Here's how the part is built. I have some questions about the finished solid (model axes, mm). A direction names the side the tool comes from. Round coordinates to 2 decimals unless told otherwise and drop trailing zeros. Order: outer loops, then holes, each group sorted by start corner. A loop starts at its lowest first (then second) coordinate and runs counter-clockwise, first axis right, second up.
Autodesk Inventor part; units mm, degrees
ref_plane "YZ Plane" through (0, 0, 0) normal (1, 0, 0) x (0, 1, 0)
ref_plane "XZ Plane" through (0, 0, 0) normal (0, 1, 0) x (-1, 0, 0)
ref_plane "XY Plane" through (0, 0, 0) normal (0, 0, 1) x (1, 0, 0)
sketch "スケッチ1" plane through (0, 0, 0) normal (1, 0, 0) x (0, 1, 0)
  circle A0 centre (0, 0) radius 9
  line L0 (50, 5.5) -> (-9, 5.5)
  line L1 (-9, 5.5) -> (-9, -13.5)
  line L2 (-9, -13.5) -> (50, -13.5)
  line L3 (50, -13.5) -> (50, 5.5)
  line L4 (50, 13.5) -> (-9, 13.5)
  line L5 (-9, 13.5) -> (-9, -13.5)
  line L6 (-9, -13.5) -> (50, -13.5)
  line L7 (50, -13.5) -> (50, 13.5)
  line L8 (-20.8, 0) -> (61.8, 0)
  point P0 (-9, 0)
  dimension "d0" = 18
  dimension "d3" = 19
  dimension "d4" = 27
extrude "押し出し1" add sketch "スケッチ1" along normal blind 1.5 contours L8 L3 L2 L1 A0 | A0 L0 L3 L8 | L1 L0 A0
sketch "スケッチ2" plane through (0, 0, 0) normal (-1, 0, 0) x (0, 0, 1)
  arc A0 (-0.2778, 12.9845) -> (-2.4907, 10.2851) centre (0, 10.5) ccw
  line L0 (-3.4833, 8.3812) -> (-3.5, 8.3716)
  line L1 (-3.5, 8.3716) -> (-3.5, 20)
  line L2 (-3.5, 20) -> (-0.5, 20)
  line L3 (-7, 20) -> (-3.5, 20)
  arc A1 (-4.5, 7.7942) -> (-5.7273, 6.9425) centre (0, 0) ccw
  line L4 (-3.5, 8.3716) -> (-4.5, 7.7942)
  arc A2 (5.5, 7.1239) -> (0, -9) centre (0, 0) ccw
  line L5 (5.5, 50) -> (5.5, 7.1239)
  line L6 (-13.5, 50) -> (5.5, 50)
  line L7 (-13.5, -9) -> (-13.5, 50)
  line L8 (0, -9) -> (-13.5, -9)
  line L9 (5.5, -9) -> (0, -9)
  line L10 (5.5, -7.1239) -> (5.5, -9)
  arc A3 (0, -9) -> (5.5, -7.1239) centre (0, 0) ccw
  arc A4 (-3.4833, 8.3812) -> (-2.4907, 10.2851) centre (-4.4833, 10.1132) ccw
  arc A5 (1.5, 18) -> (-0.5, 20) centre (-0.5, 18) ccw
  line L11 (1.5, 18) -> (1.5, 14.9721)
  arc A6 (-0.2778, 12.9845) -> (1.5, 14.9721) centre (-0.5, 14.9721) ccw
  line L12 (-9, 8.4853) -> (-9, 18)
  arc A7 (-7, 20) -> (-9, 18) centre (-7, 18) ccw
  arc A8 (-9, 8.4853) -> (-5.7273, 6.9425) centre (-7, 8.4853) ccw
  point P0 (-4.5, 7.7942)
  point P1 (-5.7273, 6.9425)
extrude "押し出し2" cut sketch "スケッチ2" against normal through all contours A6 L11 A5 L2 L3 A7 L12 A8 A2 L8 L7 L6 L5 L4 L0 A4 A0 | A3 L10 L9
sketch "スケッチ3" plane through (0, 0, 0) normal (-1, 0, 0) x (0, 0, 1)
  line L0 (-3.5, 20) -> (-3.5, 8.3716)
  line L1 (-4.5, 7.7942) -> (-3.4833, 8.3812)
  arc A0 (-0.2778, 12.9845) -> (-2.4907, 10.2851) centre (0, 10.5) ccw
  line L2 (-0.5, 20) -> (-7, 20)
  arc A1 (-4.5, 7.7942) -> (-5.7273, 6.9425) centre (0, 0) ccw
  line L3 (-3.5, 20) -> (-2.5, 20)
  line L4 (-2.5, 20) -> (-2.5, 8.3716)
  line L5 (-2.5, 8.3716) -> (-3.5, 8.3716)
  line L6 (-3.5, 8.3716) -> (-3.5, 20)
  arc A2 (-3.4833, 8.3812) -> (-2.4907, 10.2851) centre (-4.4833, 10.1132) ccw
  arc A3 (-0.2778, 12.9845) -> (1.5, 14.9721) centre (-0.5, 14.9721) ccw
  line L7 (1.5, 14.9721) -> (1.5, 18)
  arc A4 (1.5, 18) -> (-0.5, 20) centre (-0.5, 18) ccw
  arc A5 (-7, 20) -> (-9, 18) centre (-7, 18) ccw
  line L8 (-9, 18) -> (-9, 8.4853)
  arc A6 (-9, 8.4853) -> (-5.7273, 6.9425) centre (-7, 8.4853) ccw
  line L9 (-2.5, 8.3716) -> (-2.5, 10.5)
  point P0 (-2.5, 9.8557)
  dimension "d7" = 1
extrude "押し出し3" add sketch "スケッチ3" along normal blind 1 contours L2 A4 L7 A3 A0 L4 | A0 A2 L4
sketch "スケッチ4" plane through (1.5, 0, 0) normal (1, 0, 0) x (0, 0, -1)
  circle A0 centre (7, 18) radius 0.8
  circle A1 centre (7, 10.5) radius 0.8
  line L0 (7, 20) -> (0.5, 20)
  arc A2 (2.4907, 10.2851) -> (0.2778, 12.9845) centre (0, 10.5) ccw
  point P0 (0, 0)
  point P1 (-1.5, 20)
  point P2 (-1.5, 12.5)
  point P3 (2.1169, 9.1701)
  dimension "d10" = 1.6
  dimension "d11" = 1.6
  dimension "d12" = 2
extrude "押し出し4" cut sketch "スケッチ4" against normal through all
properties part number "toe_springjoint_cover_upper_left"
1. If we section it at D-D, the plane z = -8: Write out the boundary of the cut face in (x, y), and give its area (3 significant figures).
Evaluation:
outline: (0, 6.75) - (1.5, 6.75) - (1.5, 19.73) - (0, 19.73) - close
area: 19.5 mm2
2. If we mould it in two halves opening along Z, with no side actions, what happens to faces 3 (the cylindrical face through (0.76, 11.04, -6.41)), 4 (the cylindrical face through (0.232, 13.624, 0.977)), 5 (the flat face through (1.5, 15, -5)), 6 (the flat face through (1, 13, -9))? For each: released by +Z, released by -Z, zero draft, split by the parting line, or undercut.
Evaluation:
face 3: undercut
face 4: released by +Z
face 5: zero draft
face 6: released by -Z
3. If we section it at B-B, the plane x = 0.45: State how many separate pieces and enclosed holes the cut face has, and give its area (3 significant figures).
Evaluation:
separate pieces: 1
enclosed holes: 2
area: 105 mm2
4. I'm going to push a flat-ended pin straight in: P1, Ø0.7, axis at x = -0.5, y = 10, coming from the -Z side. Where does the tip first touch, or does it pass through?
Evaluation:
P1: stops at z = -2.5
5. I need wall thicknesses on probe 1 along Y at (x, z) = (0.65, -7); probe 2 along X at (y, z) = (13, -3.25); probe 3 along Z at (x, y) = (1.1, 17.5). Which ranges of each line are inside material? Lowest first, please.
Evaluation:
probe 1: y = 6.49 to 9.7, 11.3 to 17.2, 18.8 to 20
probe 2: x = 0 to 1.5
probe 3: z = -9 to -7.62, -6.38 to 1.5
6. On a 3-axis mill with a long thin cutter (end or side, diameter ignored), from which of +Z, -Z, +X, -X, +Y, -Y can I reach the whole of each face in a straight line? I mean faces 1 (the cylindrical face through (0.51, 9.404, -2.613)), 2 (the flat face through (-0.5, 15.3, -2.5)). Say none if no direction works.
Evaluation:
face 1: +Z, +X, -X
face 2: -Z, -X, +Y, -Y
7. If we section it at C-C, the plane y = 14.25: Write out the boundary of the cut face in (x, z), and give its area (3 significant figures).
Evaluation:
outline: (-1, -2.5) - (0, -2.5) - (0, -9) - (1.5, -9) - (1.5, 1.37) - (-1, 1.37) - close
area: 19.4 mm2
